The model under review builds one solid part; all positions refer to its coordinate system, in mm. A direction names the side the tool comes from. Round coordinates to 2 decimals unless told otherwise and drop trailing zeros. Loops run counter-clockwise (first coordinate to the right, second up) from the corner with the lowest first, then second, coordinate; pieces in that order, holes last. Notation, with made-up numbers: (15.25, 17.25) -> (41.25, 17.25) arc R27 ccw to (41.25, 38.25) -> close; hole circle Ø3 at (-36, 78.5). An arc over 180 degrees is marked (long way). Write each question's results on one line, items separated by ' | '. Start each with the question number.
Item 1: For L1, parallel to Z at x = 24, y = -23.5; L2, parallel to Z at x = 36, y = -19; L3, parallel to Y at x = 8.5, z = 1.75, list the stretches that pass through material, from the lowest coordinate up. Write a range as from..to.
Item 2: We need section B-B (x = 106). Give the boundary of the cut face in (y, z), and give its area (3 significant figures).
Item 3: Clearance check with flat-ended pins moving along their axes: pin 1 Ø2 at (x, z) = (26.5, -8.5) entering from -Y; pin 2 Ø1 at (x, z) = (19.5, -5.5) entering from +Y; pin 3 Ø6 at (x, y) = (87, -16) entering from -Z. State where each tip first meets the part, or that it passes through.
Item 4: Mouldability with a two-part tool opening along Z and no side actions: class faces 3 (the flat face through (61, -20, 3)), 4 (the flat face through (60.639, -15.573, -10.603)), 5 (the flat face through (0, -20, -8)) as pulls with the +Z half, pulls with the -Z half, needs draft (parallel to the pull), parting line crosses it, or undercut.
Item 5: We need section C-C (z = -10.25). Give the boundary of the cut face in (x, y).
Item 6: We need section A-A (y = -23). Give the boundary of the cut face in (x, z).
Item 7: Tool access review of faces 1 (the flat face through (61, -16, 0)), 2 (the flat face through (61, 0, 1)): name each direction out of +Z, -Z, +X, -X, +Y, -Y from which nothing blocks a thin tool from reaching the whole face with its end or side.
from build123d import *

# Parameters (mm, degrees)
F0_W     = 35
F0_H     = 3
F1_DEPTH = 123
F3_DEPTH = 123


with BuildPart() as f1:
    # F0 (on Right) → F1 (new body)
    with BuildSketch(Plane.YZ):
        with Locations((-17.5, 1.5)):
            Rectangle(F0_W, F0_H)
    extrude(amount=F1_DEPTH)

    # F2 (on face) → F3 (join, through all)
    with BuildSketch(Plane(origin=(0, 0, 0), x_dir=(0, -1, 0), z_dir=(-1, 0, 0))):
        Polygon((39.284444, 3), (35, 3), (0, -21.507264), (1.409539, -23.520294), (35, 0), align=None)
        Polygon((35, 0), (30.715556, 0), (0, -21.507264), (1.409539, -23.520294), align=None)
    extrude(amount=-F3_DEPTH)


solid = f1.part
Here are the results:
1) L1: z = -8.05..-5.05, 0..3 | L2: z = -11.2..-8.2, 0..3 | L3: y = -37.5..0
2) outline: (-39.28, 3) -> (-1.41, -23.52) -> (0, -21.51) -> (-30.72, 0) -> (0, 0) -> (0, 3) -> close | area: 208 mm2
3) pin 1: stops at y = -24.29 | pin 2: stops at y = -22.15 | pin 3: stops at z = -15.4
4) face 3: pulls with the +Z half | face 4: undercut | face 5: needs draft
5) outline: (0, -20.36) -> (123, -20.36) -> (123, -16.08) -> (0, -16.08) -> close
6) outline: (0, -8.4) -> (123, -8.4) -> (123, -5.4) -> (0, -5.4) -> close; (0, 0) -> (123, 0) -> (123, 3) -> (0, 3) -> close
7) face 1: +X, -X, +Y | face 2: +Z, -Z, +X, -X, +Y
